from build123d import *

# Parameters (mm, degrees)
F1_DEPTH = 31.75
F2_W     = 19.05
F2_H     = 12.7
F3_DEPTH = 35.053
F5_DEPTH = 35.053


with BuildPart() as f1:
    # F0 (on Front) → F1 (new body)
    with BuildSketch(Plane.XZ):
        Polygon((0, 12.7), (0, 0), (47.752, 0), (56.636066, 22.352), (91.434066, 22.352), (91.434066, 35.052), (46.984066, 35.052), (38.1, 12.7), align=None)
    extrude(amount=F1_DEPTH)

    # F2 (on face) → F3 (cut, through all)
    with BuildSketch(Plane.XY.offset(35.052)):
        with Locations((81.909066, -15.875)):
            Rectangle(F2_W, F2_H)
    extrude(amount=-F3_DEPTH, mode=Mode.SUBTRACT)

    # F4 (on face) → F5 (cut, through all)
    with BuildSketch(Plane(origin=(0, 0, 0), x_dir=(1, 0, 0), z_dir=(0, 0, -1))):
        with BuildLine():
            ThreePointArc((11.176, 15.875), (19.05, 8.001), (26.924, 15.875))
            ThreePointArc((26.924, 15.875), (19.05, 23.749), (11.176, 15.875))
        make_face()
    extrude(amount=-F5_DEPTH, mode=Mode.SUBTRACT)


solid = f1.part
Read the model definition and answer for the solid it produces. Units are mm, in the model's axes. A direction names the side the tool comes from. Coordinates: 2 decimals unless noted, no trailing zeros. Loops run counter-clockwise (first coordinate to the right, second up) from the corner with the lowest first, then second, coordinate; pieces in that order, holes last. Notation, with made-up numbers: (-12, -31) -> (-6, -31) arc R16 cw to (-6, -20) -> close; hole circle Ø9 at (66.25, -4.5). An arc over 180 degrees is marked (long way). Write item = value, one per line. Start each with the question number.
1) Find the intervals of material crossed by L1, parallel to Y at x = 19, z = 7; L2, parallel to Z at x = 83.5, y = -7; L3, parallel to Z at x = 4, y = -23.5, in increasing order. Write a range as from..to.
2) The part is cut by section B-B, the plane y = -5. Determine the outline of the cut face in (x, z).
3) The part is cut by section A-A, the plane x = 19.05. Determine the outline of the cut face in (y, z), plus the area to 3 significant figures.
4) The part is cut by section D-D, the plane y = -21. Determine the outline of the cut face in (x, z).
5) For faces 1 (the face through (91.434, -27, 29)), 2 (the face through (24, -23, 12.7)), 3 (the face through (45, 0, 18)), 4 (the face through (82, -9.525, 29)), 5 (the face through (70, -16, 22.352)), determine the directions among +Z, -Z, +X, -X, +Y, -Y from which every point of the face is accessible in a straight line to the end or side of a thin tool.
6) The mould has two halves that part along X. Classify faces 6 (the face through (12.801, -11.084, 6.261)), 7 (the face through (52.13, -15.65, 11.02)), 8 (the face through (29, -16, 0)): pulls with the +X half, pulls with the -X half, needs draft (parallel to the pull), parting line crosses it, or undercut.
7) Given P1, Ø14, axis at x = 19.05, y = -15.875, coming from the -Z side; P2, Ø12, axis at y = -21, z = 28, coming from the +X side; P3, Ø1.5, axis at y = -17, z = 30, coming from the -X side; P4, Ø9.5, axis at x = 71, y = -16, coming from the -Z side, each flat-ended and moving along its own axis, determine where each tip first touches the part or whether it passes through.
8) The part is cut by section C-C, the plane z = 31.5. Determine the outline of the cut face in (x, y) (3 decimals), plus the area to 3 significant figures.
Result:
q1.L1 = -31.75..-23.75, -8..0
q1.L2 = 22.35..35.05
q1.L3 = 0..12.7
q2.outline = (0, 0) -> (47.75, 0) -> (56.64, 22.35) -> (91.43, 22.35) -> (91.43, 35.05) -> (46.98, 35.05) -> (38.1, 12.7) -> (0, 12.7) -> close
q3.outline = (-31.75, 0) -> (-23.75, 0) -> (-23.75, 12.7) -> (-31.75, 12.7) -> close; (-8, 0) -> (0, 0) -> (0, 12.7) -> (-8, 12.7) -> close
q3.area = 203 mm²
q4.outline = (0, 0) -> (13.07, 0) -> (13.07, 12.7) -> (0, 12.7) -> close; (25.03, 0) -> (47.75, 0) -> (56.64, 22.35) -> (72.38, 22.35) -> (72.38, 35.05) -> (46.98, 35.05) -> (38.1, 12.7) -> (25.03, 12.7) -> close
q5.face_1 = +Z, -Z, +X, +Y, -Y
q5.face_2 = +Z, -X, +Y, -Y
q5.face_3 = +Z, -Z, +X, -X, +Y
q5.face_4 = +Z, -Z, +X
q5.face_5 = -Z, +X, +Y, -Y
q6.face_6 = undercut
q6.face_7 = pulls with the +X half
q6.face_8 = needs draft
q7.P1 = through
q7.P2 = 91.43
q7.P3 = 44.68
q7.P4 = 22.35
q8.outline = (45.572, -31.75) -> (91.434, -31.75) -> (91.434, -22.225) -> (72.384, -22.225) -> (72.384, -9.525) -> (91.434, -9.525) -> (91.434, 0) -> (45.572, 0) -> close
q8.area = 1,210 mm²
